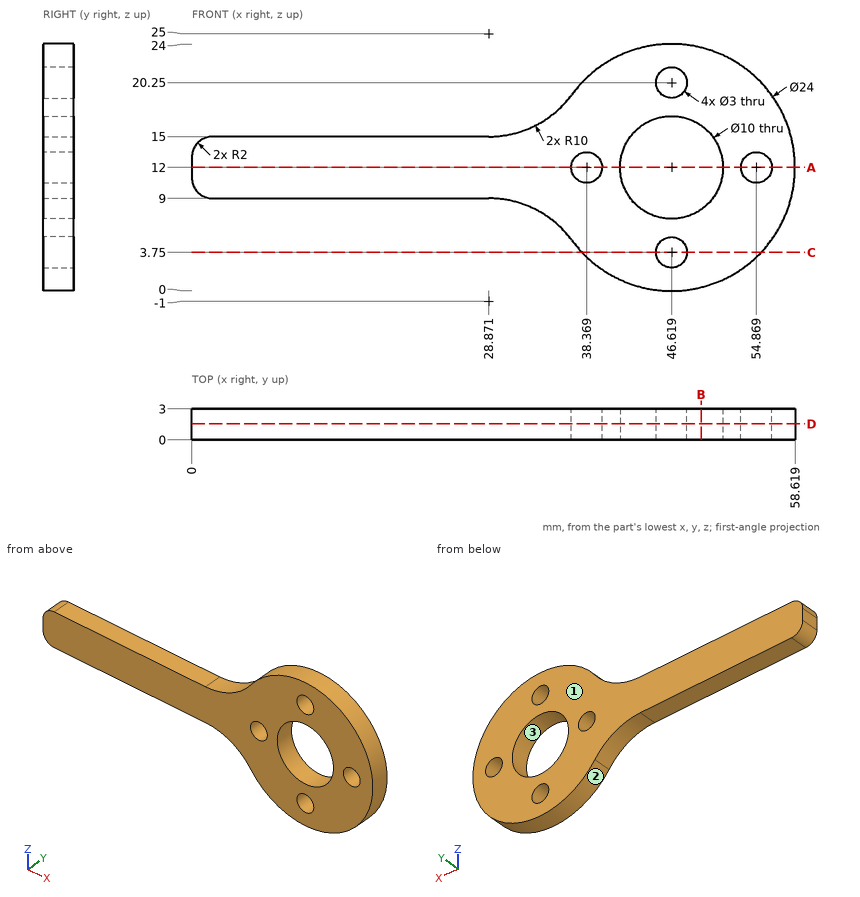
Job drawing, mm, ordinate dimensions from the low corner. One solid piece. Coordinates: 2 decimals unless noted, no trailing zeros. Order: outer loops, then holes, each group sorted by start corner. A loop starts at its lowest first (then second) coordinate and runs counter-clockwise, first axis right, second up. Notation, with made-up numbers: M 56,28 L 66,28 A24 ccw 66,58 Z; hole C 37,87 d8. An arc over 180 degrees is marked long. Return JSON: item names as keys, results as strings.
1. Drill centre lines: probe 1 along Z at (x, y) = (12, 0.75); probe 2 along X at (y, z) = (1.25, 20) (1 decimal); probe 3 along Z at (x, y) = (54, 1.9). Where is each one in solid material? Low to high.
Ans:
{"probe 1": "9 to 15", "probe 2": "37.7 to 45.1, 48.1 to 55.6", "probe 3": "2.54 to 10.78, 13.22 to 21.46"}
2. Pull direction X, two halves, no side cores. Call the marked faces 1, 2 and 3: +X half, -X half, draft (parallel to the pull), parting line (faces both ways), or undercut.
Ans:
{"face 1": "draft", "face 2": "parting line", "face 3": "undercut"}
3. Flat gauge pin, fed straight in: pin 1 (1.5 mm diameter, centred on x = 21, y = 1, fed in from +Z). Where does the tip first touch, or does it go through?
Ans:
{"pin 1": "z = 15"}
4. Saw through at C-C (z = 3.75). Give the cut face in (x, y) (1 decimal), and give its area (3 significant figures).
Ans:
{"outline": "M 37.9,0 L 45.1,0 L 45.1,3 L 37.9,3 Z; M 48.1,0 L 55.3,0 L 55.3,3 L 48.1,3 Z", "area": "43.3 mm^2"}
5. Saw through at A-A (z = 12). Give the cut face in (x, y).
Ans:
{"outline": "M 0,0 L 36.87,0 L 36.87,3 L 0,3 Z; M 39.87,0 L 41.62,0 L 41.62,3 L 39.87,3 Z; M 51.62,0 L 53.37,0 L 53.37,3 L 51.62,3 Z; M 56.37,0 L 58.62,0 L 58.62,3 L 56.37,3 Z"}
6. Saw through at D-D (y = 1.55). Give the cut face in (x, z).
Ans:
{"outline": "M 0,11 A2 ccw 2,9 L 28.87,9 A10 cw 36.94,4.91 A12 ccw long 36.94,19.09 A10 cw 28.87,15 L 2,15 A2 ccw 0,13 Z; hole C 38.37,12 d3; hole C 46.62,12 d10; hole C 46.62,3.75 d3; hole C 46.62,20.25 d3; hole C 54.87,12 d3"}
7. Saw through at B-B (x = 49.5). Give the cut face in (y, z), and give its area (3 significant figures).
Ans:
{"outline": "M 0,0.35 L 3,0.35 L 3,7.91 L 0,7.91 Z; M 0,16.09 L 3,16.09 L 3,23.65 L 0,23.65 Z", "area": "45.4 mm^2"}
